Geometry: final body of the model. Coordinates: model frame, mm. Give positions to 0.01 mm unless a question says otherwise; leave off trailing zeros. Write each loop counter-clockwise with the first axis right and the second up, starting at its lowest first coordinate (ties: lowest second). Pieces come first, ordered by that corner, then holes.
Q1. Cut plane B-B on x = -25.4. Return the cut outline in (y, z) (3 decimals), plus the area to 3 significant figures.
Q2. Cut plane C-C on z = -144. Return the cut outline in (x, y) (3 decimals).
Q3. Draft query along X for faces 1 (the face through (75.502, -31.742, 1.565)), 2 (the face through (104.731, 231.8, -125.603)), 3 (the face through (-101.6, -314, -172)). Return one class per face: pulls with the +X half, pulls with the -X half, needs draft (parallel to the pull), parting line crosses it, or undercut.
Q4. Pin query (flat end, axial travel): pin 1 (17 mm diameter, centred on x = 43, y = 8, fed in from -Z). Return the tip coordinate at first contact, or that it passes through.
Q5. Cut plane D-D on y = -351. Return the cut outline in (x, z) (3 decimals).
Q6. Cut plane A-A on z = -38.5. Return the cut outline in (x, y) (3 decimals).
```python
from build123d import *

# Parameters (mm, degrees)
F2_DEPTH = 101.6
F3_DEPTH = 95.25
F5_DEPTH = 107.95
F6_DEPTH = 101.6
F7_DEPTH = 3.175


with BuildPart() as f2:
    # F1 (on Right) → F2 (new body)
    with BuildSketch(Plane.YZ):
        Polygon((-457.2, -254), (0, 0), (0, 3.175), (-457.2, -250.825), align=None)
    extrude(amount=-F2_DEPTH)

    # F1 (on Right) → F3 (cut)
    with BuildSketch(Plane.YZ):
        Polygon((-457.2, -254), (0, 0), (0, 3.175), (-457.2, -250.825), align=None)
    extrude(amount=-F3_DEPTH, mode=Mode.SUBTRACT)



with BuildPart() as f5:
    # F4 (on Right) → F5 (new body)
    with BuildSketch(Plane.YZ):
        Polygon((0, 3.175), (0, 0), (457.2, -254), (457.2, -250.825), align=None)
    extrude(amount=F5_DEPTH)

    # F4 (on Right) → F6 (cut)
    with BuildSketch(Plane.YZ):
        Polygon((0, 3.175), (0, 0), (457.2, -254), (457.2, -250.825), align=None)
    extrude(amount=F6_DEPTH, mode=Mode.SUBTRACT)


with BuildPart() as f2_1:
    add(f2.part)

    add(f5.part)  # F7 merges F5
    # F0 (on Top) → F7 (join)
    with BuildSketch(Plane.XY):
        with BuildLine():
            ThreePointArc((0, 0), (-25.4, -25.4), (-50.8, 0))
            ThreePointArc((-50.8, 0), (-76.2, 25.4), (-101.6, 0))
            Line((-101.6, 0), (-95.25, 0))
            ThreePointArc((-95.25, 0), (-76.2, 19.05), (-57.15, 0))
            ThreePointArc((-57.15, 0), (-25.4, -31.75), (6.35, 0))
            ThreePointArc((6.35, 0), (25.4, 19.05), (44.45, 0))
            ThreePointArc((44.45, 0), (76.2, -31.75), (107.95, 0))
            Line((107.95, 0), (101.6, 0))
            ThreePointArc((101.6, 0), (76.2, -25.4), (50.8, 0))
            ThreePointArc((50.8, 0), (25.4, 25.4), (0, 0))
        make_face()
    extrude(amount=F7_DEPTH)


solid = f2_1.part
```
Data:
1. outline: (-31.75, 0) - (-25.4, 0) - (-25.4, 3.175) - (-31.75, 3.175) - close
1. area: 20.2 mm2
2. outline: (-101.6, -264.915) - (-95.25, -264.915) - (-95.25, -259.2) - (-101.6, -259.2) - close; (101.6, 259.2) - (107.95, 259.2) - (107.95, 264.915) - (101.6, 264.915) - close
3. face 1: undercut
3. face 2: needs draft
3. face 3: pulls with the -X half
4. pin 1: stops at z = 0
5. outline: (-101.6, -195) - (-95.25, -195) - (-95.25, -191.825) - (-101.6, -191.825) - close
6. outline: (-101.6, -75.015) - (-95.25, -75.015) - (-95.25, -69.3) - (-101.6, -69.3) - close; (101.6, 69.3) - (107.95, 69.3) - (107.95, 75.015) - (101.6, 75.015) - close
